Autodesk Inventor part; units mm, degrees
ref_plane "YZ Plane" through (0, 0, 0) normal (1, 0, 0) x (0, 1, 0)
ref_plane "XZ Plane" through (0, 0, 0) normal (0, 1, 0) x (-1, 0, 0)
ref_plane "XY Plane" through (0, 0, 0) normal (0, 0, 1) x (1, 0, 0)
sketch "Sketch1" plane through (0, 0, 0) normal (0, 1, 0) x (-1, 0, 0)
  line L0 (-100, 55) -> (100, 55)
  line L1 (100, 55) -> (100, -55)
  line L2 (100, -55) -> (-100, -55)
  line L3 (-100, -55) -> (-100, 55)
  line L4 (-100, 55) -> (100, -55) construction
  line L5 (100, 55) -> (-100, -55) construction
  point P0 (0, 0)
  dimension "d0" = 200
  dimension "d1" = 110
extrude "Extrusion1" add sketch "Sketch1" along normal blind 3
sketch "Sketch2" plane through (0, 3, 0) normal (0, 1, 0) x (1, 0, 0)
  line L0 (-100, -55) -> (100, -55) construction
  line L1 (100, -55) -> (100, -35) construction
  line L2 (100, -55) -> (100, 55) construction
  line L3 (100, -35) -> (80, -35) construction
  line L4 (80, -35) -> (37, -35) construction
  line L5 (80, -35) -> (123, -35) construction
  line L6 (37, -35) -> (-6, -35) construction
  line L7 (-6, -35) -> (-6, -15) construction
  line L8 (-6, -15) -> (-6, 5) construction
  line L9 (-6, 5) -> (37, 5) construction
  circle A0 centre (80, -35) radius 1.25
  circle A1 centre (37, -35) radius 1.25
  circle A2 centre (-6, -35) radius 1.25
  circle A3 centre (-6, -15) radius 1.25
  circle A4 centre (-6, 5) radius 1.25
  circle A5 centre (37, 5) radius 1.25
  line L10 (37, 5) -> (80, 5) construction
  line L11 (37, 5) -> (80, 5) construction
  line L12 (80, 5) -> (80, -15) construction
  circle A6 centre (80, 5) radius 1.25
  circle A7 centre (80, -15) radius 1.25
  point P0 (0, 0)
  dimension "d4" = 20
  dimension "d5" = 20
  dimension "d6" = 90
  dimension "d7" = 43
  dimension "d8" = 180
  dimension "d9" = 43
  dimension "d10" = 180
  dimension "d11" = 20
  dimension "d12" = 20
  dimension "d13" = 43
  dimension "d14" = 2.5
  dimension "d15" = 2.5
  dimension "d16" = 2.5
  dimension "d17" = 2.5
  dimension "d18" = 2.5
  dimension "d19" = 2.5
  dimension "d24" = 43
  dimension "d25" = 0
  dimension "d26" = 20
  dimension "d27" = 90
  dimension "d28" = 2.5
  dimension "d29" = 2.5
extrude "Extrusion2" cut sketch "Sketch2" against normal blind 3
sketch "Sketch3" plane through (0, 3, 0) normal (0, 1, 0) x (1, 0, 0)
  line L0 (-100, -55) -> (-100, 55) construction
  line L1 (-100, -55) -> (-100, -45) construction
  line L2 (-100, -45) -> (-90, -45) construction
  circle A0 centre (-90, -45) radius 2.25
  line L3 (-90, -45) -> (-90, 45) construction
  line L4 (100, -55) -> (-100, -55) construction
  line L5 (-90, -45) -> (0, -45) construction
  line L6 (-90, 45) -> (90, 45) construction
  line L7 (90, 45) -> (90, -45) construction
  circle A1 centre (-90, 45) radius 2.25
  circle A2 centre (90, 45) radius 2.25
  circle A3 centre (90, -45) radius 2.25
  line L8 (90, -45) -> (63, -45) construction
  line L9 (-90, -45) -> (-63, -45) construction
  line L10 (-90, 45) -> (-63, 45) construction
  line L11 (90, 45) -> (63, 45) construction
  circle A4 centre (63, 45) radius 2.25
  circle A5 centre (63, -45) radius 2.25
  circle A6 centre (-63, -45) radius 2.25
  circle A7 centre (-63, 45) radius 2.25
  point P0 (0, 0)
  dimension "d32" = 10
  dimension "d33" = 10
  dimension "d34" = 4.5
  dimension "d35" = 90
  dimension "d36" = 90
  dimension "d37" = 180
  dimension "d38" = 90
  dimension "d39" = 90
  dimension "d40" = 4.5
  dimension "d41" = 4.5
  dimension "d42" = 4.5
  dimension "d45" = 27
  dimension "d46" = 27
  dimension "d47" = 4.5
  dimension "d48" = 4.5
  dimension "d49" = 4.5
  dimension "d50" = 4.5
  dimension "d64" = 27
  dimension "d65" = 27
extrude "Extrusion4" cut sketch "Sketch3" against normal up to surface (3 mm away)
sketch "Sketch4" plane through (0, 0, 0) normal (0, -1, 0) x (1, 0, 0)
  circle A0 centre (-90, 45) radius 2.25 construction
  circle A1 centre (-63, 45) radius 2.25 construction
  circle A2 centre (-63, -45) radius 2.25 construction
  circle A3 centre (63, 45) radius 2.25 construction
  circle A4 centre (90, 45) radius 2.25 construction
  circle A5 centre (-90, -45) radius 2.25 construction
  circle A6 centre (-90, 45) radius 2.25 construction
  circle A7 centre (90, -45) radius 2.25 construction
  circle A8 centre (63, -45) radius 2.25 construction
  circle A9 centre (80, -5) radius 1.25 construction
  circle A10 centre (-6, -5) radius 1.25 construction
  circle A11 centre (-6, 35) radius 1.25 construction
  circle A12 centre (80, 35) radius 1.25 construction
  circle A13 centre (37, 35) radius 1.25 construction
  circle A14 centre (-6, 15) radius 1.25 construction
  circle A15 centre (37, -5) radius 1.25 construction
  circle A16 centre (80, 15) radius 1.25 construction
  line L0 (100, 55) -> (-100, 55) construction
  line L1 (-100, 55) -> (-100, -55) construction
  line L2 (-100, -55) -> (100, -55) construction
  line L3 (100, -55) -> (100, 55) construction
  circle A17 centre (-63, 45) radius 2.25 construction
  circle A18 centre (-63, -45) radius 2.25 construction
  circle A19 centre (63, 45) radius 2.25 construction
  circle A20 centre (90, 45) radius 2.25 construction
  circle A21 centre (-90, -45) radius 2.25 construction
  circle A22 centre (-90, 45) radius 2.25 construction
  circle A23 centre (90, -45) radius 2.25 construction
  circle A24 centre (63, -45) radius 2.25 construction
  circle A25 centre (80, -5) radius 1.25 construction
  circle A26 centre (-6, -5) radius 1.25 construction
  circle A27 centre (-6, 35) radius 1.25 construction
  circle A28 centre (80, 35) radius 1.25 construction
  circle A29 centre (37, 35) radius 1.25 construction
  circle A30 centre (-6, 15) radius 1.25 construction
  circle A31 centre (37, -5) radius 1.25 construction
  circle A32 centre (80, 15) radius 1.25 construction
  line L4 (100, 55) -> (-100, 55) construction
  line L5 (-100, 55) -> (-100, -55) construction
  line L6 (-100, -55) -> (100, -55) construction
  line L7 (100, -55) -> (100, 55) construction
  line L8 (-90, 45) -> (-90, 0) construction
  line L9 (-90, 45) -> (-45, 45) construction
  circle A33 centre (-90, 0) radius 1.25
  line L10 (-90, 0) -> (-90, 25) construction
  line L11 (-90, 0) -> (-90, -25) construction
  circle A34 centre (-90, 25) radius 1.25
  circle A35 centre (-90, -25) radius 1.25
  point P0 (0, 0)
  dimension "d55" = 45
  dimension "d56" = 90
  dimension "d57" = 2.5
  dimension "d58" = 25
  dimension "d59" = 25
  dimension "d60" = 2.5
  dimension "d61" = 2.5
  dimension "d90" = 10
extrude "Extrusion5" cut sketch "Sketch4" against normal up to surface (3 mm away)
sketch "Sketch5" plane through (0, 3, 0) normal (0, 1, 0) x (1, 0, 0)
  line L0 (-100, -55) -> (100, -55)
  line L1 (-71.5, -55) -> (-43.5, -55) construction
  line L2 (-72, -27) -> (-72, 27)
  line L3 (-72, 27) -> (-45, 27)
  line L4 (-72, 27) -> (-45, 27) construction
  line L5 (-72, -27) -> (-18, -27)
  line L6 (-72, -27) -> (-18, -27) construction
  circle A0 centre (-72, -27) radius 1.5
  circle A1 centre (-18, -27) radius 1.5
  circle A2 centre (-45, 27) radius 1.5
  circle A3 centre (-90, -25) radius 1.25
  circle A4 centre (-90, 25) radius 1.25
  circle A5 centre (-90, 0) radius 1.25
  circle A6 centre (-63, -45) radius 2.25
  circle A7 centre (-63, 45) radius 2.25
  circle A8 centre (63, -45) radius 2.25
  circle A9 centre (90, -45) radius 2.25
  circle A10 centre (-90, 45) radius 2.25
  circle A11 centre (-90, -45) radius 2.25
  circle A12 centre (90, 45) radius 2.25
  circle A13 centre (63, 45) radius 2.25
  circle A14 centre (80, 5) radius 1.25
  circle A15 centre (-6, 5) radius 1.25
  circle A16 centre (-6, -35) radius 1.25
  circle A17 centre (80, -35) radius 1.25
  circle A18 centre (37, -35) radius 1.25
  circle A19 centre (-6, -15) radius 1.25
  circle A20 centre (37, 5) radius 1.25
  circle A21 centre (80, -15) radius 1.25
  line L7 (-100, -55) -> (100, -55)
  line L8 (100, -55) -> (100, 55)
  line L9 (100, 55) -> (-100, 55)
  line L10 (-100, 55) -> (-100, -55)
  line L11 (-45, 27) -> (-18, 27)
  line L12 (-45, 27) -> (-18, 27) construction
  circle A22 centre (-18, 27) radius 1.5
  point P0 (0, 0)
  dimension "d70" = 54
  dimension "d72" = 27
  dimension "d73" = 0
  dimension "d74" = 54
  dimension "d75" = 0
  dimension "d76" = 3
  dimension "d77" = 3
  dimension "d79" = 3
  dimension "d82" = 12
  dimension "d83" = 28
  dimension "d84" = 90
  dimension "d85" = 27
  dimension "d86" = 0
  dimension "d87" = 3
extrude "Extrusion8" cut sketch "Sketch5" against normal blind 10 contours L5 A0 L2 | L2 A0 L5 | A22 | A2 L11 L3 | L3 L11 A2 | A1
properties part number "foot"
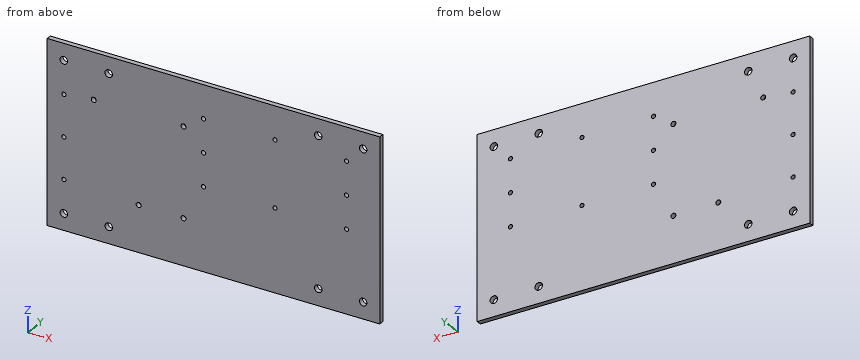
Geometry: final body of the model. Coordinates: model frame, mm. Coordinates: 2 decimals unless noted, no trailing zeros. Order: outer loops, then holes, each group sorted by start corner. A loop starts at its lowest first (then second) coordinate and runs counter-clockwise, first axis right, second up. Notation, with made-up numbers: (-29.75, -13.5) -> (-0.75, -13.5) arc R24 cw to (-0.75, 1.5) -> close; hole circle Ø7 at (85, 31.25). An arc over 180 degrees is marked (long way). Write item = value, one per line.
(1) Cut plane B-B on z = 45. Return loops of the section in (x, y).
Solved:
outline = (-100, 0) -> (-92.25, 0) -> (-92.25, 3) -> (-100, 3) -> close; (-87.75, 0) -> (-65.25, 0) -> (-65.25, 3) -> (-87.75, 3) -> close; (-60.75, 0) -> (60.75, 0) -> (60.75, 3) -> (-60.75, 3) -> close; (65.25, 0) -> (87.75, 0) -> (87.75, 3) -> (65.25, 3) -> close; (92.25, 0) -> (100, 0) -> (100, 3) -> (92.25, 3) -> close
(2) Pin query (flat end, axial travel): pin 1 Ø2 at (x, z) = (-90, 0) entering from -Y. Return the tip coordinate at first contact, or that it passes through.
Solved:
pin_1 = through
(3) Line query: line 1 (X direction, y = 1.15, z = 15); line 2 (Z direction, x = 80, y = 0.85); line 3 (X direction, y = 0.2, z = -5). Output: solid intervals per line, ascending.
Solved:
line_1 = -100 to -7.25, -4.75 to 78.75, 81.25 to 100
line_2 = -55 to -6.25, -3.75 to 13.75, 16.25 to 33.75, 36.25 to 55
line_3 = -100 to -7.25, -4.75 to 35.75, 38.25 to 78.75, 81.25 to 100
(4) Cut plane A-A on x = 90. Return loops of the section in (y, z), plus the area to 3 significant figures.
Solved:
outline = (0, -55) -> (3, -55) -> (3, -47.25) -> (0, -47.25) -> close; (0, -42.75) -> (3, -42.75) -> (3, 42.75) -> (0, 42.75) -> close; (0, 47.25) -> (3, 47.25) -> (3, 55) -> (0, 55) -> close
area = 303 mm²
